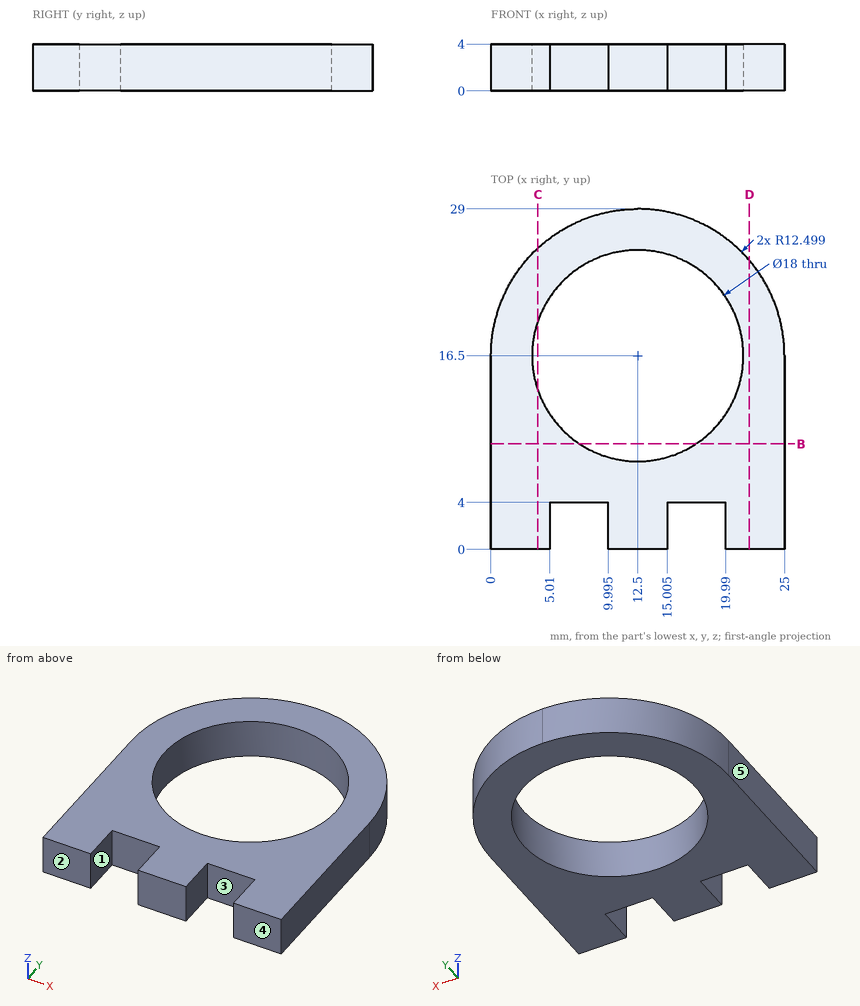
Verification items for this drawing (mm, ordinates from the low corner). A direction names the side the tool comes from. Give positions to 0.01 mm unless a question says otherwise; leave off trailing zeros. Loops run counter-clockwise (first coordinate to the right, second up) from the corner with the lowest first, then second, coordinate; pieces in that order, holes last. Notation, with made-up numbers: M 66.5,77 L 120.5,77 A26 ccw 120.5,104 Z; hole C -12.5,-30 d1. An arc over 180 degrees is marked long. Return JSON: item names as keys, results as strings. Group by question number.
1. Go/stop test with flat-tipped pins: pin 1 (14.5 mm diameter, centred on x = 12.5, y = 16.5, fed in from -Z); pin 2 (2 mm diameter, centred on x = 16.5, z = 2.5, fed in from -Y). Record where each tip stops, or that it passes through.
2. Cross-section at B-B on y = 9. Record the boundary of the cut face in (x, z) (1 decimal).
3. Cross-section at C-C on x = 4. Record the boundary of the cut face in (y, z).
4. Thickness scan on L1, parallel to Y at x = 12.5, z = 2.6; L2, parallel to X at y = 16.25, z = 3.15; L3, parallel to X at y = 9, z = 2.6 (1 decimal). Record the ranges inside material, lowest first.
5. Cross-section at D-D on x = 22. Record the boundary of the cut face in (y, z) (1 decimal), plus the area to 3 significant figures.
6. Tool access check on the marked faces 1 and 2. Record the directions out of +Z, -Z, +X, -X, +Y, -Y that give a thin tool (end or side, any length) a straight path to the whole face; none if there is none.
7. Mould release check, pull along X, two halves, no side actions. Record for the marked faces 3, 4 and 5: released by +X, released by -X, zero draft, split by the parting line, or undercut.
Return value:
{
 "1": {"pin 1": "through", "pin 2": "y = 4"},
 "2": {"outline": "M 0,0 L 7.5,0 L 7.5,4 L 0,4 Z; M 17.5,0 L 25,0 L 25,4 L 17.5,4 Z"},
 "3": {"outline": "M 0,0 L 13.54,0 L 13.54,4 L 0,4 Z; M 19.46,0 L 25.67,0 L 25.67,4 L 19.46,4 Z"},
 "4": {"L1": "0 to 7.5, 25.5 to 29", "L2": "0 to 3.5, 21.5 to 25", "L3": "0 to 7.5, 17.5 to 25"},
 "5": {"outline": "M 0,0 L 24.6,0 L 24.6,4 L 0,4 Z", "area": "98.5 mm^2"},
 "6": {"face 1": "+Z, -Z, -Y", "face 2": "+Z, -Z, +X, -X, -Y"},
 "7": {"face 3": "undercut", "face 4": "zero draft", "face 5": "released by -X"}
}
